Geometry: see drawing. Coordinates: mm, zero at the bounding-box minimum. A direction names the side the tool comes from. Give positions to 0.01 mm unless a question says otherwise; leave off trailing zeros. Loops run counter-clockwise (first coordinate to the right, second up) from the corner with the lowest first, then second, coordinate; pieces in that order, holes last. Notation, with made-up numbers: M 6,15 L 40,15 A20 cw 40,36 Z; hole C 56.5,41 d7. An arc over 180 degrees is marked long. Answer in a Markdown table with one row per item.
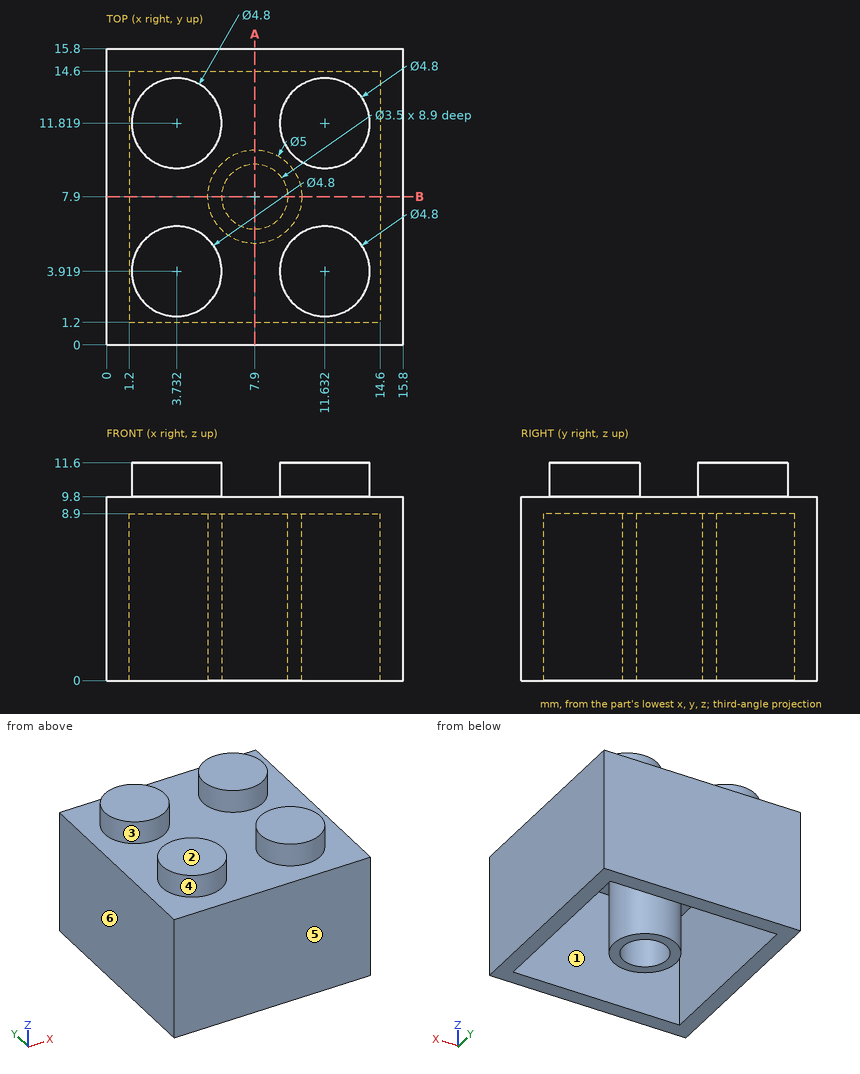
1) Set-up query: the marked faces 1, 2 and 3. Return all of +Z, -Z, +X, -X, +Y, -Y with unobstructed straight access to the full face (end or side cutting, diameter ignored); none if empty.
Reply:
| item | result |
|---|---|
| face 1 | -Z |
| face 2 | +Z, +X, -X, +Y, -Y |
| face 3 | +Z |
2) Material intervals for L1, parallel to X at y = 7.9, z = 5; L2, parallel to Y at x = 9.5, z = 8.5, sorted ascending.
Reply:
| item | result |
|---|---|
| L1 | x = 0 to 1.2, 5.4 to 6.15, 9.65 to 10.4, 14.6 to 15.8 |
| L2 | y = 0 to 1.2, 5.98 to 7.19, 8.61 to 9.82, 14.6 to 15.8 |
3) Pull-direction query (Y, two-part tool) for the marked faces 4, 5 and 6; classes: released by +Y, released by -Y, zero draft, split by the parting line, or undercut.
Reply:
| item | result |
|---|---|
| face 4 | undercut |
| face 5 | released by -Y |
| face 6 | zero draft |
4) Section A-A, the plane x = 7.9. Return loops of the section in (y, z).
Reply:
| item | result |
|---|---|
| outline | M 0,0 L 1.2,0 L 1.2,8.9 L 5.4,8.9 L 5.4,0 L 6.15,0 L 6.15,8.9 L 9.65,8.9 L 9.65,0 L 10.4,0 L 10.4,8.9 L 14.6,8.9 L 14.6,0 L 15.8,0 L 15.8,9.8 L 0,9.8 Z |
5) Pin query (flat end, axial travel): pin 1 Ø5.5 at (x, y) = (7.9, 7.9) entering from -Z; pin 2 Ø1.5 at (x, y) = (8.5, 7) entering from +Z. Return the tip coordinate at first contact, or that it passes through.
Reply:
| item | result |
|---|---|
| pin 1 | stops at z = 0 |
| pin 2 | stops at z = 9.8 |
